from build123d import *

# Parameters (mm, degrees)
F0_R     = 3.175
F1_DEPTH = 38.1
F2_R     = 9.525
F3_DEPTH = 6.35
F4_R     = 9.525
F5_DEPTH = 6.35


with BuildPart() as f1:
    # F0 (on Top) → F1 (new body, symmetric)
    with BuildSketch(Plane.XY):
        Circle(F0_R)
    extrude(amount=F1_DEPTH, both=True)

    # F2 (on face) → F3 (join)
    with BuildSketch(Plane(origin=(0, 0, -38.1), x_dir=(1, 0, 0), z_dir=(0, 0, -1))):
        Circle(F2_R)
    extrude(amount=-F3_DEPTH)

    # F4 (on face) → F5 (join)
    with BuildSketch(Plane.XY.offset(38.1)):
        Circle(F4_R)
    extrude(amount=-F5_DEPTH)


solid = f1.part
Input: part model. Units: mm. Frame: model coordinates. A direction names the side the tool comes from. Coordinates: 2 decimals unless noted, no trailing zeros. Order: outer loops, then holes, each group sorted by start corner. A loop starts at its lowest first (then second) coordinate and runs counter-clockwise, first axis right, second up. Notation, with made-up numbers: M 6,33.25 L 37,33.25 A18 ccw 37,47.25 Z; hole C 53,-39.75 d4. An arc over 180 degrees is marked long. Answer in a Markdown table with one row per item.
(1) Section query B-B, the plane x = -4.5. Output: boundary loops of the cut face in (y, z).
Numbers:
| item | result |
|---|---|
| outline | M -8.39,-38.1 L 8.39,-38.1 L 8.39,-31.75 L -8.39,-31.75 Z; M -8.39,31.75 L 8.39,31.75 L 8.39,38.1 L -8.39,38.1 Z |
(2) Contact query for flat-ended pins moving along their axis: pin 1 Ø10 at (y, z) = (4.5, -7) entering from -X (3 decimals); pin 2 Ø8 at (y, z) = (7.5, 2.5) entering from -X; pin 3 Ø8 at (x, z) = (5.5, 27) entering from -Y. Output: stop coordinate, or through.
Numbers:
| item | result |
|---|---|
| pin 1 | stops at x = -3.175 |
| pin 2 | passes through |
| pin 3 | stops at y = -2.8 |
(3) Section query C-C, the plane y = 4.25. Output: boundary loops of the cut face in (x, z).
Numbers:
| item | result |
|---|---|
| outline | M -8.52,-38.1 L 8.52,-38.1 L 8.52,-31.75 L -8.52,-31.75 Z; M -8.52,31.75 L 8.52,31.75 L 8.52,38.1 L -8.52,38.1 Z |
(4) Material intervals for line 1 (Z direction, x = -7, y = -2.5); line 2 (Y direction, x = 2.75, z = -29); line 3 (Y direction, x = -2.25, z = -3), sorted ascending. Write a range as [from, to].
Numbers:
| item | result |
|---|---|
| line 1 | z = [-38.1, -31.75], [31.75, 38.1] |
| line 2 | y = [-1.59, 1.59] |
| line 3 | y = [-2.24, 2.24] |
(5) Section query A-A, the plane y = 0. Output: boundary loops of the cut face in (x, z) (3 decimals).
Numbers:
| item | result |
|---|---|
| outline | M -9.525,-38.1 L 9.525,-38.1 L 9.525,-31.75 L 3.175,-31.75 L 3.175,31.75 L 9.525,31.75 L 9.525,38.1 L -9.525,38.1 L -9.525,31.75 L -3.175,31.75 L -3.175,-31.75 L -9.525,-31.75 Z |
(6) Access query for faces 1 (the flat face through (4, 0, 31.75)), 2 (the cylindrical face through (-7.559, -5.796, 34.969)). Directions: +Z, -Z, +X, -X, +Y, -Y. A direction counts if a zero-diameter tool reaches every point of the face in a straight line with its end or side. Return the directions, or none.
Numbers:
| item | result |
|---|---|
| face 1 | none |
| face 2 | +Z, -Z |
(7) Draft query along Z for faces 3 (the flat face through (4, 0, -31.75)), 4 (the cylindrical face through (-7.559, 5.796, -34.969)), 5 (the flat face through (0, 0, 38.1)). Return one class per face: pulls with the +Z half, pulls with the -Z half, needs draft (parallel to the pull), parting line crosses it, or undercut.
Numbers:
| item | result |
|---|---|
| face 3 | undercut |
| face 4 | needs draft |
| face 5 | pulls with the +Z half |
